For this review, take the finished solid that the model builds, in its own axes (mm). Give positions to 0.01 mm unless a question says otherwise; leave off trailing zeros. Write each loop counter-clockwise with the first axis right and the second up, starting at its lowest first coordinate (ties: lowest second). Pieces come first, ordered by that corner, then holes. Notation, with made-up numbers: M -9,-4.5 L 18,-4.5 A23 cw 18,23.5 Z; hole C 48,81 d3. An arc over 180 degrees is marked long. Write item = value, one per line.
```python
from build123d import *

# Parameters (mm, degrees)
SKETCH1_W               = 336.55
SKETCH1_H               = 158.75
BOSS_EXTRUDE1_DEPTH     = 5.588
F_1_4_CLEARANCE_HOLE1_D = 6.7564
F_6_CLEARANCE_HOLE1_D   = 3.7973
F_6_CLEARANCE_HOLE2_D   = 3.7973
CUT_EXTRUDE1_REACH      = 188.14
F_10_CLEARANCE_HOLE1_D  = 5.1054
CUT_EXTRUDE2_REACH      = 188.14
F_10_CLEARANCE_HOLE3_D  = 5.1054
F_10_CLEARANCE_HOLE2_D  = 5.1054
F_10_CLEARANCE_HOLE4_D  = 5.1054
CUT_EXTRUDE3_REACH      = 188.14
SKETCH24_R              = 2.5527


with BuildPart() as part:
    # Sketch1 → Boss-Extrude1 (new body)
    with BuildSketch(Plane.XY):
        Rectangle(SKETCH1_W, SKETCH1_H)
    extrude(amount=BOSS_EXTRUDE1_DEPTH)

    # 1/4 Clearance Hole1 (through all)
    with Locations(Plane(origin=(0, 0, 0), x_dir=(-1, 0, 0), z_dir=(0, 0, -1))):
        with Locations((-158.75, 69.85), (158.75, -63.5), (-158.75, -63.5), (158.75, 69.85)):
            Hole(F_1_4_CLEARANCE_HOLE1_D / 2)

    # #6 Clearance Hole1 (through all)
    with Locations(Plane(origin=(0, 0, 0), x_dir=(-1, 0, 0), z_dir=(0, 0, -1))):
        with Locations((-155.575, 41.275), (-155.575, -6.985), (-78.105, 41.275)):
            Hole(F_6_CLEARANCE_HOLE1_D / 2)

    # #6 Clearance Hole2 (through all)
    with Locations(Plane(origin=(0, 0, 0), x_dir=(-1, 0, 0), z_dir=(0, 0, -1))):
        with Locations((-142.875, 15.875), (-84.875, -33.125), (-142.875, -33.125), (-84.875, 15.875)):
            Hole(F_6_CLEARANCE_HOLE2_D / 2)

    # Sketch11 → Cut-Extrude1 (cut, up to next)
    with BuildSketch(Plane(origin=(0, 0, 0), x_dir=(-1, 0, 0), z_dir=(0, 0, -1)), mode=Mode.PRIVATE) as cut_extrude1_sk1:
        with BuildLine():
            Line((-13.335, 19.05), (19.685, 19.05))
            ThreePointArc((19.685, 19.05), (21.481051224, 18.306051224), (22.225, 16.51))
            Line((22.225, 16.51), (22.225, -51.435))
            ThreePointArc((22.225, -51.435), (21.481051224, -53.231051224), (19.685, -53.975))
            Line((19.685, -53.975), (-13.335, -53.975))
            ThreePointArc((-13.335, -53.975), (-15.131051224, -53.231051224), (-15.875, -51.435))
            Line((-15.875, -51.435), (-15.875, 16.51))
            ThreePointArc((-15.875, 16.51), (-15.131051224, 18.306051224), (-13.335, 19.05))
        make_face()
    cut_extrude1_tool1 = extrude(cut_extrude1_sk1.sketch, amount=-CUT_EXTRUDE1_REACH, mode=Mode.PRIVATE) & part.part
    add(cut_extrude1_tool1.solids().sort_by_distance((-3.175, -17.4625, 0))[0], mode=Mode.SUBTRACT)

    # #10 Clearance Hole1 (through all)
    with Locations(Plane(origin=(0, 0, 0), x_dir=(-1, 0, 0), z_dir=(0, 0, -1))):
        with Locations((3.175, 24.60625), (3.175, -59.53125)):
            Hole(F_10_CLEARANCE_HOLE1_D / 2)

    # Sketch15 → Cut-Extrude2 (cut, up to next)
    with BuildSketch(Plane(origin=(0, 0, 0), x_dir=(-1, 0, 0), z_dir=(0, 0, -1)), mode=Mode.PRIVATE) as cut_extrude2_sk1:
        with BuildLine():
            Line((-60.325, 53.975), (-34.925, 53.975))
            ThreePointArc((-34.925, 53.975), (-30.434871939, 52.115128061), (-28.575, 47.625))
            Line((-28.575, 47.625), (-28.575, -47.625))
            ThreePointArc((-28.575, -47.625), (-30.434871939, -52.115128061), (-34.925, -53.975))
            Line((-34.925, -53.975), (-60.325, -53.975))
            ThreePointArc((-60.325, -53.975), (-64.815128061, -52.115128061), (-66.675, -47.625))
            Line((-66.675, -47.625), (-66.675, 47.625))
            ThreePointArc((-66.675, 47.625), (-64.815128061, 52.115128061), (-60.325, 53.975))
        make_face()
    cut_extrude2_tool1 = extrude(cut_extrude2_sk1.sketch, amount=-CUT_EXTRUDE2_REACH, mode=Mode.PRIVATE) & part.part
    add(cut_extrude2_tool1.solids().sort_by_distance((47.625, 0, 0))[0], mode=Mode.SUBTRACT)

    # #10 Clearance Hole3 (through all)
    with Locations(Plane(origin=(0, 0, 0), x_dir=(-1, 0, 0), z_dir=(0, 0, -1))):
        with Locations((131.2799, 30.7848), (131.2799, -34.925), (141.7701, 30.7848), (141.7701, -34.925)):
            Hole(F_10_CLEARANCE_HOLE3_D / 2)

    # #10 Clearance Hole2 (through all)
    with Locations(Plane(origin=(0, 0, 0), x_dir=(-1, 0, 0), z_dir=(0, 0, -1))):
        with Locations((-47.625, 73.025), (53.975, 60.325), (-47.625, 60.325), (53.975, 73.025)):
            Hole(F_10_CLEARANCE_HOLE2_D / 2)

    # #10 Clearance Hole4 (through all)
    with Locations(Plane(origin=(0, 0, 0), x_dir=(-1, 0, 0), z_dir=(0, 0, -1))):
        with Locations((44.323, -41.275), (92.075, -41.275)):
            Hole(F_10_CLEARANCE_HOLE4_D / 2)

    # Sketch24 → Cut-Extrude3 (cut, up to next)
    with BuildSketch(Plane(origin=(0, 0, 0), x_dir=(-1, 0, 0), z_dir=(0, 0, -1)), mode=Mode.PRIVATE) as cut_extrude3_sk1:
        with Locations((110.175, 53.975)):
            Circle(SKETCH24_R)
    cut_extrude3_tool1 = extrude(cut_extrude3_sk1.sketch, amount=-CUT_EXTRUDE3_REACH, mode=Mode.PRIVATE) & part.part
    # Sketch24 → Cut-Extrude3 (cut, up to next)
    with BuildSketch(Plane(origin=(0, 0, 0), x_dir=(-1, 0, 0), z_dir=(0, 0, -1)), mode=Mode.PRIVATE) as cut_extrude3_sk2:
        with Locations((150.175, 53.975)):
            Circle(SKETCH24_R)
    cut_extrude3_tool2 = extrude(cut_extrude3_sk2.sketch, amount=-CUT_EXTRUDE3_REACH, mode=Mode.PRIVATE) & part.part
    # Sketch24 → Cut-Extrude3 (cut, up to next)
    with BuildSketch(Plane(origin=(0, 0, 0), x_dir=(-1, 0, 0), z_dir=(0, 0, -1)), mode=Mode.PRIVATE) as cut_extrude3_sk3:
        with BuildLine():
            Line((120.025, 65.125), (140.325, 65.125))
            ThreePointArc((140.325, 65.125), (143.860533906, 63.660533906), (145.325, 60.125))
            Line((145.325, 60.125), (145.325, 47.825))
            ThreePointArc((145.325, 47.825), (143.860533906, 44.289466094), (140.325, 42.825))
            Line((140.325, 42.825), (120.025, 42.825))
            ThreePointArc((120.025, 42.825), (116.489466094, 44.289466094), (115.025, 47.825))
            Line((115.025, 47.825), (115.025, 60.125))
            ThreePointArc((115.025, 60.125), (116.489466094, 63.660533906), (120.025, 65.125))
        make_face()
    cut_extrude3_tool3 = extrude(cut_extrude3_sk3.sketch, amount=-CUT_EXTRUDE3_REACH, mode=Mode.PRIVATE) & part.part
    add(cut_extrude3_tool1.solids().sort_by_distance((-110.175, 53.975, 0))[0], mode=Mode.SUBTRACT)
    add(cut_extrude3_tool2.solids().sort_by_distance((-150.175, 53.975, 0))[0], mode=Mode.SUBTRACT)
    add(cut_extrude3_tool3.solids().sort_by_distance((-130.175, 53.975, 0))[0], mode=Mode.SUBTRACT)


solid = part.part
```
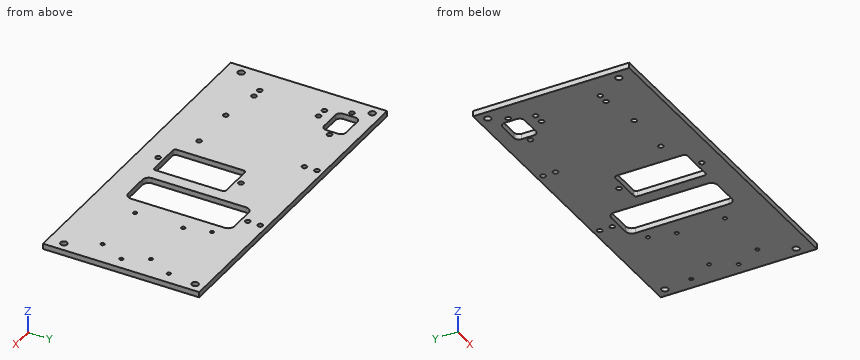
1. Insertion check: P1, Ø4, axis at x = -53.975, y = 73.025, coming from the -Z side. The pin has a flat end and moves straight along its axis. Give the tip position at first contact, or say it passes through.
Responses:
P1 = through
2. For line 1 along X through (y, z) = (-12, 2.9) (3 decimals); line 2 along Y through (x, z) = (158.75, 1.65) (3 decimals); line 3 along Y through (x, z) = (34.5, 2.4) (3 decimals), list the stretches that pass through material, from the lowest coordinate up. Write a range as from..to.
Responses:
line_1 = -168.275..-22.225, 15.875..28.575, 66.675..168.275
line_2 = -79.375..-66.878, -60.122..66.472, 73.228..79.375
line_3 = -79.375..-53.961, 53.961..79.375
3. We need section C-C, the plane z = 1.35. Count the separate pieces of the cut face and the enclosed holes in it, then the cut area to 3 significant figures.
Responses:
separate_pieces = 1
enclosed_holes = 28
area = 45,400 mm2
4. We need section A-A, the plane y = -15. Write out the cut boundary in (x, z) (3 decimals), then the cut area to 3 significant figures.
Responses:
outline = M -168.275,0 L -22.225,0 L -22.225,5.588 L -168.275,5.588 Z; M 15.875,0 L 28.575,0 L 28.575,5.588 L 15.875,5.588 Z; M 66.675,0 L 168.275,0 L 168.275,5.588 L 66.675,5.588 Z
area = 1,450 mm2
5. We need section B-B, the plane x = -158.75. Write out the cut boundary in (y, z) (3 decimals).
Responses:
outline = M -79.375,0 L -66.878,0 L -66.878,5.588 L -79.375,5.588 Z; M -60.122,0 L 66.472,0 L 66.472,5.588 L -60.122,5.588 Z; M 73.228,0 L 79.375,0 L 79.375,5.588 L 73.228,5.588 Z
